```python
from build123d import *

# Parameters (mm, degrees)
BOSS_EXTRUDE1_DEPTH = 5.08
SKETCH3_W           = 5.08
SKETCH3_H           = 5.08
CUT_EXTRUDE1_DEPTH  = 5.08
CUT_EXTRUDE2_DEPTH  = 5.08


with BuildPart() as part:
    # Sketch1 → Boss-Extrude1 (new body)
    with BuildSketch(Plane(origin=(0, 0, 0), x_dir=(1, 0, 0), z_dir=(0, 1, 0))):
        Polygon((53.32, 0), (26.66, 46.17647453), (-26.66, 46.17647453), (-53.32, 0), (-26.66, -46.17647453), (26.66, -46.17647453), align=None)
    extrude(amount=BOSS_EXTRUDE1_DEPTH)

    # Sketch3 → Cut-Extrude1 (cut)
    with BuildSketch(Plane(origin=(0, 5.08, 0), x_dir=(1, 0, 0), z_dir=(0, 1, 0))):
        with Locations((-17.78, 43.63647453)):
            Rectangle(SKETCH3_W, SKETCH3_H)
        with Locations((7.62, 43.63647453)):
            Rectangle(SKETCH3_W, SKETCH3_H)
        with Locations((17.78, 43.63647453)):
            Rectangle(SKETCH3_W, SKETCH3_H)
        with Locations((-7.62, 43.63647453)):
            Rectangle(SKETCH3_W, SKETCH3_H)
        Polygon((29.83, 40.68587347), (25.430590949, 38.14587347), (27.970590949, 33.746464419), (32.37, 36.286464419), align=None)
        Polygon((42.53, 18.688828214), (45.07, 14.289419162), (40.670590949, 11.749419162), (38.130590949, 16.148828214), align=None)
        Polygon((47.61, 9.890010111), (50.15, 5.49060106), (45.750590949, 2.95060106), (43.210590949, 7.350010111), align=None)
        Polygon((34.91, 31.887055367), (30.510590949, 29.347055367), (33.050590949, 24.947646316), (37.45, 27.487646316), align=None)
        Polygon((50.15, -5.49060106), (45.750590949, -2.95060106), (43.210590949, -7.350010111), (47.61, -9.890010111), align=None)
        Polygon((37.45, -27.487646316), (34.91, -31.887055367), (30.510590949, -29.347055367), (33.050590949, -24.947646316), align=None)
        Polygon((32.37, -36.286464419), (29.83, -40.68587347), (25.430590949, -38.14587347), (27.970590949, -33.746464419), align=None)
        Polygon((45.07, -14.289419162), (40.670590949, -11.749419162), (38.130590949, -16.148828214), (42.53, -18.688828214), align=None)
        with Locations((17.78, -43.63647453)):
            Rectangle(SKETCH3_W, SKETCH3_H)
        with Locations((-7.62, -43.63647453)):
            Rectangle(SKETCH3_W, SKETCH3_H)
        with Locations((-17.78, -43.63647453)):
            Rectangle(SKETCH3_W, SKETCH3_H)
        with Locations((7.62, -43.63647453)):
            Rectangle(SKETCH3_W, SKETCH3_H)
        Polygon((-29.83, -40.68587347), (-25.430590949, -38.14587347), (-27.970590949, -33.746464419), (-32.37, -36.286464419), align=None)
        Polygon((-42.53, -18.688828214), (-45.07, -14.289419162), (-40.670590949, -11.749419162), (-38.130590949, -16.148828214), align=None)
        Polygon((-47.61, -9.890010111), (-50.15, -5.49060106), (-45.750590949, -2.95060106), (-43.210590949, -7.350010111), align=None)
        Polygon((-34.91, -31.887055367), (-30.510590949, -29.347055367), (-33.050590949, -24.947646316), (-37.45, -27.487646316), align=None)
        Polygon((-50.15, 5.49060106), (-45.750590949, 2.95060106), (-43.210590949, 7.350010111), (-47.61, 9.890010111), align=None)
        Polygon((-37.45, 27.487646316), (-34.91, 31.887055367), (-30.510590949, 29.347055367), (-33.050590949, 24.947646316), align=None)
        Polygon((-32.37, 36.286464419), (-29.83, 40.68587347), (-25.430590949, 38.14587347), (-27.970590949, 33.746464419), align=None)
        Polygon((-45.07, 14.289419162), (-40.670590949, 11.749419162), (-38.130590949, 16.148828214), (-42.53, 18.688828214), align=None)
    extrude(amount=-CUT_EXTRUDE1_DEPTH, mode=Mode.SUBTRACT)

    # Sketch4 → Cut-Extrude2 (cut)
    with BuildSketch(Plane(origin=(0, 5.08, 0), x_dir=(1, 0, 0), z_dir=(0, 1, 0))):
        Polygon((0, 7.62), (2.54, 7.62), (2.54, 2.54), (7.62, 2.54), (7.62, 0), (7.62, -2.54), (2.54, -2.54), (2.54, -7.62), (0, -7.62), (-2.54, -7.62), (-2.54, -2.54), (-7.62, -2.54), (-7.62, 0), (-7.62, 2.54), (-2.54, 2.54), (-2.54, 7.62), align=None)
    extrude(amount=-CUT_EXTRUDE2_DEPTH, mode=Mode.SUBTRACT)


solid = part.part
```
Verification items for the finished model (mm, model axes). A direction names the side the tool comes from. Round coordinates to 2 decimals unless told otherwise and drop trailing zeros. Order: outer loops, then holes, each group sorted by start corner. A loop starts at its lowest first (then second) coordinate and runs counter-clockwise, first axis right, second up. Notation, with made-up numbers: (60.5, 74) - (95.5, 74) arc R9 ccw to (95.5, 84) - close; hole circle Ø9 at (15, 5.5). An arc over 180 degrees is marked (long way). Use CSV: the item, a comma, the result in double quotes.
(1) Thickness scan on probe 1 along Z at (x, y) = (-34, 3.15); probe 2 along Z at (x, y) = (40, 0.3); probe 3 along Z at (x, y) = (-6, 2.4). Record the ranges inside material, lowest first. Write a range as from..to.
Entries:
probe 1,"-33.46..-31.36, -25.5..25.5, 31.36..33.46"
probe 2,"-23.07..-17.23, -12.91..12.91, 17.23..23.07"
probe 3,"-41.1..-2.54, 2.54..41.1"
(2) Access from +Z, -Z, +X, -X, +Y, -Y to the whole of each face (thin tool, end or side, straight path). Record for faces 5 (the face through (-35.22, 2.58, 26.2)), 6 (the face through (-10.16, 3, 44)), 7 (the face through (-5.08, 3, -44)).
Entries:
face 5,"+Y, -Y"
face 6,"+Z, +Y, -Y"
face 7,"-Z, +Y, -Y"
(3) Gauge pin test, flat ends, axial feed: pin 1 Ø1.5 at (y, z) = (2, 43) entering from +X; pin 2 Ø1 at (y, z) = (3.5, 3.5) entering from -X; pin 3 Ø2 at (x, y) = (-41, 1) entering from +Z; pin 4 Ø1 at (x, z) = (-37, -11.5) entering from -Y. Record the tip position at first contact, or that the pin passes through.
Entries:
pin 1,"x = 28.93"
pin 2,"x = -51.59"
pin 3,"z = 23.07"
pin 4,"y = 0"
(4) Section check B-B on z = -22. Record the boundary of the cut face in (x, y).
Entries:
outline,"(-40.62, 0) - (40.62, 0) - (40.62, 5.08) - (-40.62, 5.08) - close"
(5) Section check A-A on x = 19. Record the boundary of the cut face in (y, z).
Entries:
outline,"(0, -41.1) - (5.08, -41.1) - (5.08, 41.1) - (0, 41.1) - close"
(6) Mould release check, pull along X, two halves, no side actions. Record for faces 1 (the face through (-35.22, 2.58, -26.2)), 2 (the face through (-13, 3, 46.176)), 3 (the face through (-46.322, 2.504, -12.121)), 4 (the face through (-5, 3, 2.54)): released by +X, released by -X, zero draft, split by the parting line, or undercut.
Entries:
face 1,"undercut"
face 2,"zero draft"
face 3,"released by -X"
face 4,"undercut"
